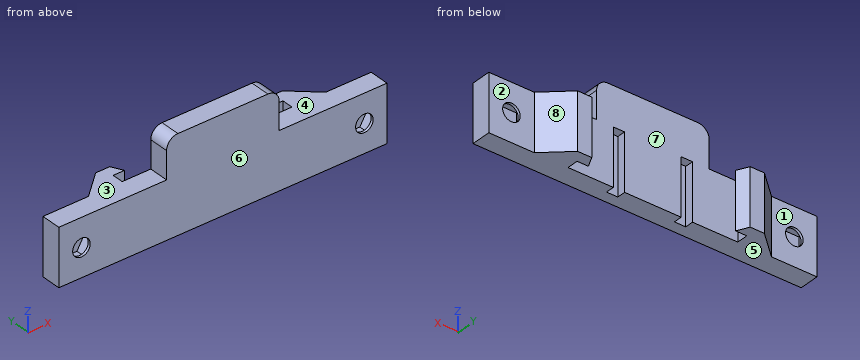
from build123d import *

# Parameters (mm, degrees)
SKETCH1_W           = 58
SKETCH1_H           = 10
BOSS_EXTRUDE1_DEPTH = 1.75
SKETCH2_R           = 1.55
CUT_EXTRUDE1_DEPTH  = 3.5
CUT_EXTRUDE2_DEPTH  = 1.3
SKETCH5_W           = 19.9
SKETCH5_H           = 23.7
BOSS_EXTRUDE2_DEPTH = 1.75
FILLET1_R           = 2
BOSS_EXTRUDE3_DEPTH = 5
SKETCH7_W           = 2
SKETCH7_H           = 10
CUT_EXTRUDE3_DEPTH  = 1.5
SKETCH8_W           = 23.808980199
SKETCH8_H           = 14.934673145
CUT_EXTRUDE4_DEPTH  = 5


with BuildPart() as part:
    # Sketch1 → Boss-Extrude1 (new, symmetric)
    with BuildSketch(Plane(origin=(0, 0, 0), x_dir=(1, 0, 0), z_dir=(0, 1, 0))):
        Rectangle(SKETCH1_W, SKETCH1_H)
    extrude(amount=BOSS_EXTRUDE1_DEPTH, both=True)

    # Sketch2 → Cut-Extrude1 (cut)
    with BuildSketch(Plane(origin=(0, 1.75, 0), x_dir=(1, 0, 0), z_dir=(0, 1, 0))):
        with Locations(Location((-25, 0, 0), (0, 0, 270))):
            Circle(SKETCH2_R)
        with Locations(Location((25, 0, 0), (0, 0, 270))):
            Circle(SKETCH2_R)
    extrude(amount=-CUT_EXTRUDE1_DEPTH, mode=Mode.SUBTRACT)

    # Sketch4 → Cut-Extrude2 (cut, symmetric)
    with BuildSketch(Plane(origin=(0, 0, 0), x_dir=(1, 0, 0), z_dir=(0, 1, 0))):
        Polygon((-28.290896534, 0), (-28.290896534, -2.85), (-26.645448267, -2.85), (-23.354551733, -2.85), (-21.709103466, -2.85), (-21.709103466, 0), (-23.354551733, 2.85), (-26.645448267, 2.85), align=None)
        Polygon((28.290896534, 0), (26.645448267, 2.85), (23.354551733, 2.85), (21.709103466, 0), (21.709103466, -2.85), (23.354551733, -2.85), (26.645448267, -2.85), (28.290896534, -2.85), align=None)
    extrude(amount=CUT_EXTRUDE2_DEPTH, both=True, mode=Mode.SUBTRACT)

    # Sketch5 → Boss-Extrude2 (add, symmetric)
    with BuildSketch(Plane(origin=(0, 0, 0), x_dir=(1, 0, 0), z_dir=(0, 1, 0))):
        Rectangle(SKETCH5_W, SKETCH5_H)
    extrude(amount=BOSS_EXTRUDE2_DEPTH, both=True)

    # Fillet1
    fillet1_edges = [part.edges().sort_by_distance(p)[0] for p in [
        (9.95, 0, 11.85),
        (-9.95, 0, 11.85),
    ]]
    fillet(fillet1_edges, radius=FILLET1_R)

    # Sketch6 → Boss-Extrude3 (add, symmetric)
    with BuildSketch(Plane.XY):
        Polygon((-20.964458506, 1.75), (-16.5, 5.75), (-14, 5.75), (-13, 3.75), (-15, 3.75), (-15, 1.75), align=None)
    boss_extrude3 = extrude(amount=BOSS_EXTRUDE3_DEPTH, both=True)

    # Mirror1: Boss-Extrude3 across plane
    add(boss_extrude3.mirror(Plane(origin=(0, 0, 0), x_dir=(0, 0, 1), z_dir=(1, 0, 0))))

    # Sketch7 → Cut-Extrude3 (cut)
    with BuildSketch(Plane(origin=(0, 1.75, 0), x_dir=(1, 0, 0), z_dir=(0, 1, 0))):
        with Locations((-6, 0)):
            Rectangle(SKETCH7_W, SKETCH7_H)
        with Locations((6, 0)):
            Rectangle(SKETCH7_W, SKETCH7_H)
    extrude(amount=-CUT_EXTRUDE3_DEPTH, mode=Mode.SUBTRACT)

    # Sketch8 → Cut-Extrude4 (cut, symmetric)
    with BuildSketch(Plane(origin=(0, 0, 0), x_dir=(1, 0, 0), z_dir=(0, 1, 0))):
        with Locations((0.433446228, 12.467336573)):
            Rectangle(SKETCH8_W, SKETCH8_H)
    extrude(amount=CUT_EXTRUDE4_DEPTH, both=True, mode=Mode.SUBTRACT)


solid = part.part
Here's how the part is built. I have some questions about the finished solid (model axes, mm). Face numbers are marked on the shaded views. A direction names the side the tool comes from. Round coordinates to 2 decimals unless told otherwise and drop trailing zeros. Loops run counter-clockwise (first coordinate to the right, second up) from the corner with the lowest first, then second, coordinate; pieces in that order, holes last. Notation, with made-up numbers: M 41.25,-17 L 77.25,-17 A16 cw 77.25,-3 Z; hole C 53.25,43 d5. An arc over 180 degrees is marked long. Write each question's results on one line, items separated by ' | '. Start each with the question number.
(1) I want a section at A-A (x = 25). Please give me the cut outline in (y, z).
(2) On a 3-axis mill with a long thin cutter (end or side, diameter ignored), from which of +Z, -Z, +X, -X, +Y, -Y can I reach the whole of each face in a straight line? I mean the marked faces 1, 2, 3, 4 and 5. Say none if no direction works.
(3) I want a section at C-C (x = 6). Please give me the cut outline in (y, z).
(4) Will these pins go through, and if not, where does the flat tip stop? P1, Ø3, axis at y = 5, z = -3, coming from the +X side; P2, Ø2, axis at x = -24.5, y = 0, coming from the +Z side; P3, Ø0.8, axis at x = -6.5, y = 1, coming from the -Z side.
(5) Thinking about a two-plate mould opening in X: for the marked faces 6, 7 and 8, which applies, pulls with the +X half, pulls with the -X half, needs draft (parallel to the pull), parting line crosses it, or undercut?
(6) I want a section at D-D (z = 7.75). Please give me the cut outline in (x, y), then the cut area to 4 significant figures.
(7) I want a section at B-B (y = -0.5). Please give me the cut outline in (x, z), then the cut area to 3 significant figures.
(8) If I drill on probe 1 along X at (y, z) = (-0.75, 0.25); probe 2 along X at (y, z) = (0.5, 0.75); probe 3 along X at (y, z) = (-1.5, 0), over which ranges is the centre line in solid material (lowest first)? Write a range as from..to.
Solved:
1) outline: M -1.75,-5 L 1.75,-5 L 1.75,-1.55 L 1.3,-1.55 L 1.3,-2.85 L -1.3,-2.85 L -1.3,-1.55 L -1.75,-1.55 Z; M -1.75,1.55 L -1.3,1.55 L -1.3,2.85 L 1.3,2.85 L 1.3,1.55 L 1.75,1.55 L 1.75,5 L -1.75,5 Z
2) face 1: +Z, -Z, -X, +Y | face 2: +Z, -Z, +X, +Y | face 3: +Z, -X, +Y, -Y | face 4: +Z, +X, +Y, -Y | face 5: -Z, +X, -X, +Y, -Y
3) outline: M -1.75,-5 L 0.25,-5 L 0.25,5 L 1.75,5 L 1.75,11.85 L -1.75,11.85 Z
4) P1: stops at x = 19.01 | P2: stops at z = 5 | P3: stops at z = 5
5) face 6: needs draft | face 7: undercut | face 8: pulls with the +X half
6) outline: M -9.95,-1.75 L 9.95,-1.75 L 9.95,1.75 L -9.95,1.75 Z | area: 69.65 mm²
7) outline: M -29,-5 L 29,-5 L 29,5 L 9.95,5 L 9.95,9.85 A2 ccw 7.95,11.85 L -7.95,11.85 A2 ccw -9.95,9.85 L -9.95,5 L -29,5 Z; hole M -28.29,0 L -26.65,-2.85 L -23.35,-2.85 L -21.71,0 L -21.71,2.85 L -28.29,2.85 Z; hole M 21.71,0 L 23.35,-2.85 L 26.65,-2.85 L 28.29,0 L 28.29,2.85 L 21.71,2.85 Z | area: 649 mm²
8) probe 1: x = -29..-28.29, -21.71..21.71, 28.29..29 | probe 2: x = -29..-28.29, -21.71..-7, -5..5, 7..21.71, 28.29..29 | probe 3: x = -29..-26.55, -23.45..23.45, 26.55..29
